Autodesk Inventor part; units mm, degrees
ref_plane "XY Plane" through (0, 0, 0) normal (0, 0, 1) x (1, 0, 0)
sketch "Sketch1" plane through (0, 0, 0) normal (0, 0, 1) x (1, 0, 0)
  line L0 (0, 0) -> (72, 0)
  line L1 (72, 0) -> (72, 47)
  line L2 (72, 47) -> (0, 47)
  line L3 (0, 47) -> (0, 0)
  circle A0 centre (3, 23.5) radius 1.65
  circle A1 centre (69, 23.5) radius 1.65
  line L4 (0, 23.5) -> (72, 23.5) construction
  circle A2 centre (18, 39.5) radius 2.2
  circle A3 centre (54, 39.5) radius 2.2
  circle A4 centre (54, 7.5) radius 2.2
  circle A5 centre (18, 7.5) radius 2.2
  line L5 (18, 39.5) -> (18, 7.5) construction
  line L6 (18, 7.5) -> (54, 7.5) construction
  line L7 (54, 7.5) -> (54, 39.5) construction
  line L8 (54, 39.5) -> (18, 39.5) construction
  line L9 (3.1536, 51.5748) -> (75.0735, 51.5748) construction
  line L10 (75.0735, 51.5748) -> (75.0735, -9.0389) construction
  line L11 (75.0735, -9.0389) -> (3.1536, -9.0389) construction
  line L12 (3.1536, -9.0389) -> (3.1536, 51.5748) construction
  circle A6 centre (10, 34) radius 6
  line L13 (36, 0) -> (36, 47)
  line L14 (9, 28.0839) -> (9, 23.5)
  line L15 (15.3327, 36.75) -> (36, 36.75)
  circle A7 centre (62, 34) radius 6
  line L16 (63, 28.0839) -> (63, 23.5)
  line L17 (56.6673, 36.75) -> (36, 36.75)
  circle A8 centre (10, 13) radius 6
  line L18 (9, 18.9161) -> (9, 23.5)
  line L19 (15.3327, 10.25) -> (36, 10.25)
  circle A9 centre (62, 13) radius 6
  line L20 (56.6673, 10.25) -> (36, 10.25)
  line L21 (63, 18.9161) -> (63, 23.5)
  line L22 (26, 10.25) -> (46, 10.25)
  line L23 (46, 10.25) -> (46, 0)
  line L24 (46, 0) -> (26, 0)
  line L25 (26, 0) -> (26, 10.25)
  point P0 (36, 39.5)
  point P1 (54, 23.5)
  dimension "d0" = 72
  dimension "d1" = 47
  dimension "d2" = 3.3
  dimension "d3" = 3.3
  dimension "d4" = 66
  dimension "d5" = 3
  dimension "d6" = 36
  dimension "d7" = 32
  dimension "d8" = 36
  dimension "d9" = 4.4
  dimension "d10" = 4.4
  dimension "d11" = 4.4
  dimension "d12" = 4.4
  dimension "d32" = 12
  dimension "d33" = 10
  dimension "d34" = 13
  dimension "d35" = 9
  dimension "d36" = 10.25
  dimension "d44" = 10
  dimension "d45" = 10
extrude "Extrusion1" add sketch "Sketch1" against normal blind 3.5 contours L3 L2 L13 L15 A6 L14 L18 A8 L19 L25 L0 | L25 L19 L13 L0 | L13 L20 L23 L0 | L2 L1 L0 L23 L20 A9 L21 L16 A7 L17 L13 | A2 | A3 | A4 | A5
extrude "Extrusion2" cut sketch "Sketch1" against normal through all draft -7 contours A2 | A3 | A4 | A5
fillet "Fillet1" radius 5 8 edges at (9, 18.9161, -1.75) (9, 28.0839, -1.75) (15.3327, 36.75, -1.75) (56.6673, 36.75, -1.75) (63, 18.9161, -1.75) (56.6673, 10.25, -1.75) (15.3327, 10.25, -1.75) (63, 28.0839, -1.75)
extrude "Extrusion3" cut sketch "Sketch1" against normal through all contours L25 L19 L13 L0 | L13 L20 L23 L0
fillet "Fillet2" radius 5 4 edges at (26, 10.25, -1.75) (46, 10.25, -1.75) (26, 0, -1.75) (46, 0, -1.75)
sketch "Sketch2" plane through (0, 0, 0) normal (0, 0, 1) x (1, 0, 0)
  arc A0 (6.7273, 18.0288) -> (9, 22.2195) centre (4, 22.2195) ccw
  arc A1 (6.7273, 18.0288) -> (14.258, 8.7727) centre (10, 13) ccw
  line L0 (9, 22.2195) -> (9, 24.7805)
  arc A2 (6.7273, 18.0288) -> (9, 22.2195) centre (4, 22.2195) ccw
  line L1 (9, 22.2195) -> (9, 14.4433) construction
  line L2 (9, 14.4433) -> (4.4748, 7.8488) construction
  arc A3 (6.7273, 18.0288) -> (14.258, 8.7727) centre (10, 13) ccw
  line L3 (4.4748, 7.8488) -> (9, 7.0839) construction
  spline S0 degree 3 poles (9, 22.2195) (9, 14.4433) (4.4748, 7.8488) (9, 7.0839) knots 1 1 1 1 2 2 2 2
  point P0 (0, 0)
  point P1 (8.9999, 7.0839)
  dimension "d50" = 1
extrude "Extrusion4" add sketch "Sketch2" against normal up to surface (3.5 mm away)
ref_plane "Work Plane1" through (3, 23.5, 0) normal (0, 1, 0) x (-1, 0, 0)
mirror "Mirror1" about plane through (3, 23.5, 0) normal (0, 1, 0) of "Extrusion4"
ref_plane "Work Plane2" through (36, 10.25, 0) normal (1, 0, 0) x (0, 1, 0)
mirror "Mirror2" about plane through (36, 10.25, 0) normal (1, 0, 0) of "Extrusion4", "Mirror1"
equation "\"d10\" = d9"
equation "\"d11\" = d9"
equation "\"d12\" = d9"
properties part number "lidar_mount_frame_lidar_lite_v3hp"
Verification items for the finished model (mm, model axes). A direction names the side the tool comes from. Coordinates: 2 decimals unless noted, no trailing zeros. Order: outer loops, then holes, each group sorted by start corner. A loop starts at its lowest first (then second) coordinate and runs counter-clockwise, first axis right, second up. Notation, with made-up numbers: (6.25, 50.5) - (39.25, 50.5) arc R33 ccw to (39.25, 85.5) - close; hole circle Ø3 at (-11, 14.5). An arc over 180 degrees is marked (long way). Return JSON: item names as keys, results as strings.
(1) Section check D-D, the plane y = 41. Give the number of separate pieces and of enclosed holes in the cut face, and give its area (3 significant figures).
Filled sheet:
{"separate pieces": "3", "enclosed holes": "0", "area": "234 mm^2"}
(2) Go/stop test with flat-tipped pins: pin 1 (3 mm diameter, centred on x = 69, y = 23.5, fed in from +Z); pin 2 (1.8 mm diameter, centred on x = 41.5, z = -1, fed in from -Y). Record where each tip stops, or that it passes through.
Filled sheet:
{"pin 1": "passes through", "pin 2": "stops at y = 36.75"}
(3) Mould release check, pull along Y, two halves, no side actions. Record for faces 3 (the conical face through (52.06, 39.59, -2.11)), 4 (the flat face through (37, 39, 0)), 5 (the cylindrical face through (2.785, 25.136, -1.726)), 6 (the cylindrical face through (48, 1, -2)): pulls with the +Y half, pulls with the -Y half, needs draft (parallel to the pull), parting line crosses it, or undercut.
Filled sheet:
{"face 3": "undercut", "face 4": "needs draft", "face 5": "undercut", "face 6": "pulls with the -Y half"}
(4) Access from +Z, -Z, +X, -X, +Y, -Y to the whole of each face (thin tool, end or side, straight path). Record for faces 1 (the flat face through (19, 10.25, -2)), 2 (the flat face through (61, 0, -2)).
Filled sheet:
{"face 1": "+Z, -Z", "face 2": "+Z, -Z, +X, -X, -Y"}
(5) Thickness scan on line 1 along Y through (x, z) = (3, -1.05); line 2 along X through (y, z) = (9, -2.65); line 3 along Y through (x, z) = (17.5, -1.75). Record the ranges inside material, lowest first.
Filled sheet:
{"line 1": "y = 0 to 21.85, 25.15 to 47", "line 2": "x = 0 to 7.03, 14.5 to 16.88, 19.12 to 24.31, 47.69 to 52.88, 55.12 to 57.5, 64.97 to 72", "line 3": "y = 0 to 5.58, 9.42 to 10.24, 36.76 to 37.58, 41.42 to 47"}
(6) Section check B-B, the plane y = 23.5. Record the cut outline in (x, z).
Filled sheet:
{"outline": "(0, -3.5) - (1.35, -3.5) - (1.35, 0) - (0, 0) - close; (4.65, -3.5) - (9, -3.5) - (9, 0) - (4.65, 0) - close; (63, -3.5) - (67.35, -3.5) - (67.35, 0) - (63, 0) - close; (70.65, -3.5) - (72, -3.5) - (72, 0) - (70.65, 0) - close"}
(7) Section check C-C, the plane x = 40.5. Record the cut outline in (y, z), and give its area (3 significant figures).
Filled sheet:
{"outline": "(36.75, -3.5) - (47, -3.5) - (47, 0) - (36.75, 0) - close", "area": "35.9 mm^2"}
(8) Section check A-A, the plane x = 3. Record the cut outline in (y, z).
Filled sheet:
{"outline": "(0, -3.5) - (21.85, -3.5) - (21.85, 0) - (0, 0) - close; (25.15, -3.5) - (47, -3.5) - (47, 0) - (25.15, 0) - close"}
